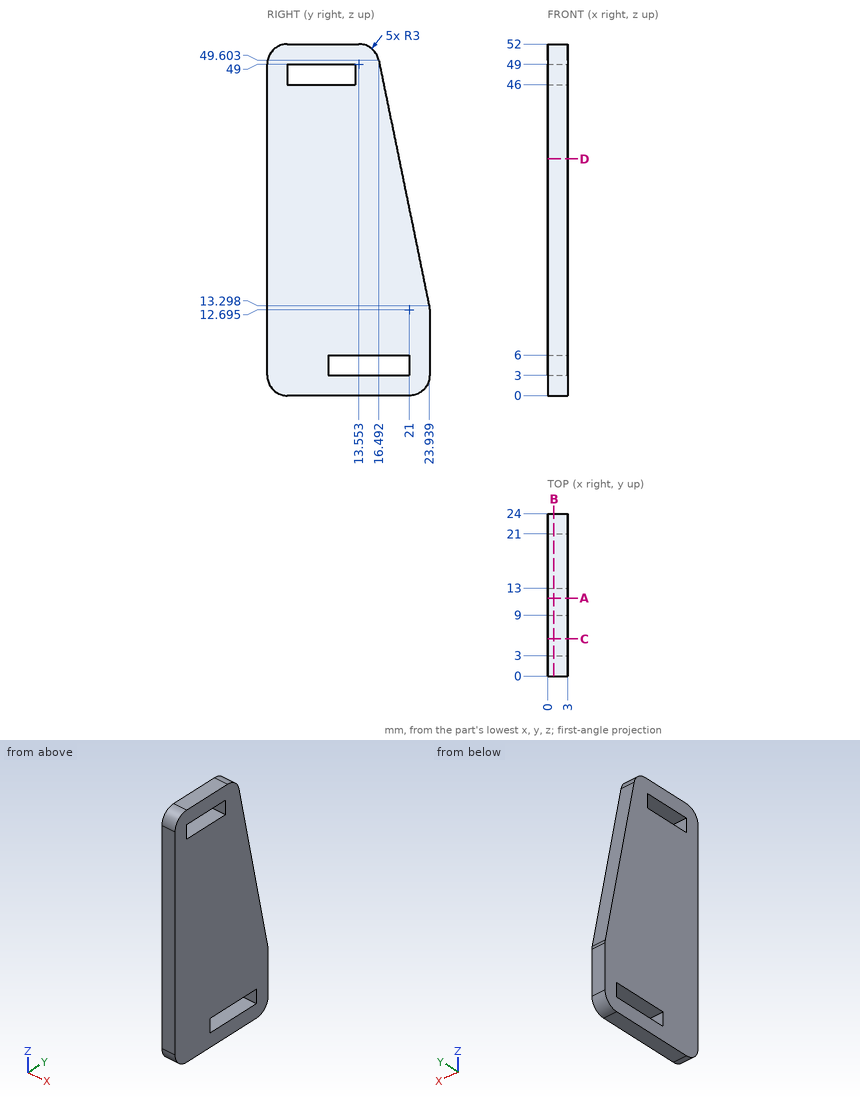
Geometry check sheet. Reference: drawing and pictorial views, mm from the part's lowest x, y, z. Round coordinates to 2 decimals unless told otherwise and drop trailing zeros. Loops run counter-clockwise (first coordinate to the right, second up) from the corner with the lowest first, then second, coordinate; pieces in that order, holes last. Notation, with made-up numbers: (-10, 62) -> (-1, 62) arc R16 cw to (-1, 92) -> close; hole circle Ø3 at (-2.5, 51). An arc over 180 degrees is marked (long way). Answer as a JSON object with one key per item and string values.
Q1. Section check C-C (y = 5.5). Record the boundary of the cut face in (x, z).
Data:
{"outline": "(0, 0) -> (3, 0) -> (3, 46) -> (0, 46) -> close; (0, 49) -> (3, 49) -> (3, 52) -> (0, 52) -> close"}
Q2. Section check B-B (x = 0.95). Record the boundary of the cut face in (y, z) (1 decimal).
Data:
{"outline": "(0, 3) arc R3 ccw to (3, 0) -> (21, 0) arc R3 ccw to (24, 3) -> (24, 12.7) arc R3 ccw to (23.9, 13.3) -> (16.5, 49.6) arc R3 ccw to (13.6, 52) -> (3, 52) arc R3 ccw to (0, 49) -> close; hole (3, 46) -> (13, 46) -> (13, 49) -> (3, 49) -> close; hole (9, 3) -> (21, 3) -> (21, 6) -> (9, 6) -> close"}
Q3. Go/stop test with a flat-tipped pin: P1, Ø3, axis at y = 2.5, z = 19, coming from the -X side. Record where the tip stops, or that it passes through.
Data:
{"P1": "stops at x = 0"}
Q4. Scan lines: line 1 (Z direction, x = 2.7, y = 11); line 2 (Z direction, x = 0.1, y = 8.25); line 3 (Y direction, x = 1.2, z = 4). Record each from-to range of solid material in increasing order. Write a range as from..to.
Data:
{"line 1": "z = 0..3, 6..46, 49..52", "line 2": "z = 0..46, 49..52", "line 3": "y = 0..9, 21..24"}
Q5. Section check D-D (z = 35). Record the boundary of the cut face in (x, y).
Data:
{"outline": "(0, 0) -> (3, 0) -> (3, 19.49) -> (0, 19.49) -> close"}
Q6. Section check A-A (y = 11.5). Record the boundary of the cut face in (x, z).
Data:
{"outline": "(0, 0) -> (3, 0) -> (3, 3) -> (0, 3) -> close; (0, 6) -> (3, 6) -> (3, 46) -> (0, 46) -> close; (0, 49) -> (3, 49) -> (3, 52) -> (0, 52) -> close"}
